from build123d import *

# Parameters (mm, degrees)
SKETCH_R        = 1.5
PAD_DEPTH       = 10
SKETCH001_R     = 4.5
POCKET_DEPTH    = 30.352032
SKETCH002_R     = 8.25
POCKET001_DEPTH = 25


with BuildPart() as part:
    # Sketch → Pad (new body)
    with BuildSketch(Plane.XY):
        with BuildLine():
            ThreePointArc((0, 70.5), (-15.559169, 68.761634), (-30.351032, 63.632263))
            Line((-30.351032, 63.632263), (-30.351032, 93.25))
            Line((-30.351032, 93.25), (0, 93.25))
            Line((0, 93.25), (0, 70.5))
        make_face()
        with Locations((-7.5, 90.25)):
            Circle(SKETCH_R, mode=Mode.SUBTRACT)
        with Locations((-22.5, 90.25)):
            Circle(SKETCH_R, mode=Mode.SUBTRACT)
    extrude(amount=PAD_DEPTH)

    # Sketch001 (on Face4 of Pad) → Pocket (cut, through all)
    with BuildSketch(Plane.YZ):
        with Locations((78.25, 0)):
            Circle(SKETCH001_R)
    extrude(amount=-POCKET_DEPTH, mode=Mode.SUBTRACT)

    # Sketch002 (on Face2 of Pocket) → Pocket001 (cut)
    with BuildSketch(Plane.YZ.offset(-2.5)):
        with Locations((78.25, 0)):
            Circle(SKETCH002_R)
    extrude(amount=-POCKET001_DEPTH, mode=Mode.SUBTRACT)


solid = part.part
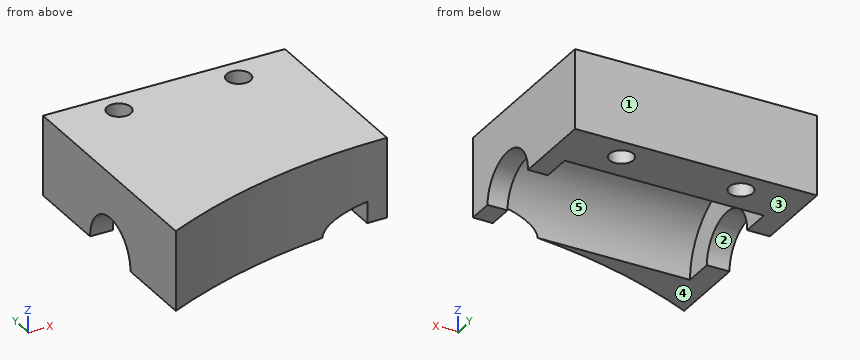
Can you work these out from the model? Positions are in its coordinate system, mm. Face numbers are marked on the shaded views. A direction names the side the tool comes from. Coordinates: 2 decimals unless noted, no trailing zeros. Write each loop counter-clockwise with the first axis right and the second up, starting at its lowest first coordinate (ties: lowest second). Pieces come first, ordered by that corner, then holes. Notation, with made-up numbers: (87.25, -20) -> (123.25, -20) arc R15 cw to (123.25, -1) -> close; hole circle Ø8 at (-17, 67). An arc over 180 degrees is marked (long way). Write each question's results on one line, items separated by ' | '. Start each with the question number.
Q1. We'd pull the mould along Y, two halves only. Please class the marked faces 1, 2 and 3: +Y half, -Y half, draft (parallel to the pull), parting line (faces both ways), or undercut.
Q2. Imagine slicing it at B-B (z = 2). Write out the boundary of the cut face in (x, y).
Q3. If I drill on probe 1 along X at (y, z) = (90.25, 4.5); probe 2 along Y at (x, z) = (-22.5, 4.25); probe 3 along Y at (x, z) = (-22.5, 5.25), over which ranges is the centre line in solid material (lowest first)?
Q4. Imagine slicing it at C-C (z = 9.25). Write out the boundary of the cut face in (x, y), then the cut area to 3 significant figures.
Q5. Imagine slicing it at A-A (x = -22.5). Write out the boundary of the cut face in (y, z), then the cut area to 3 significant figures.
Q6. On a 3-axis mill with a long thin cutter (end or side, diameter ignored), from which of +Z, -Z, +X, -X, +Y, -Y can I reach the whole of each face in a straight line? I mean the marked faces 4 and 5. Say none if no direction works.
Q7. Imagine slicing it at D-D (y = 72). Write out the boundary of the cut face in (x, z).
Q8. I'm going to push a flat-ended pin straight in: pin 1 (2 mm diameter, centred on x = -14, z = 2.5, fed in from -Y). Where does the tip first touch, or does it pass through?
Taken from the geometry:
1) face 1: +Y half | face 2: undercut | face 3: draft
2) outline: (-30.35, 63.63) arc R70.5 cw to (-5.98, 70.25) -> (-27.5, 70.25) -> (-27.5, 74.22) -> (-30.35, 74.22) -> close; (-30.35, 82.28) -> (-27.5, 82.28) -> (-27.5, 86.25) -> (-2.5, 86.25) -> (-2.5, 82.28) -> (0, 82.28) -> (0, 93.25) -> (-30.35, 93.25) -> close; (-2.5, 70.46) arc R70.5 cw to (0, 70.5) -> (0, 74.22) -> (-2.5, 74.22) -> close; hole circle Ø3 at (-22.5, 90.25); hole circle Ø3 at (-7.5, 90.25)
3) probe 1: x = -30.35 to -24, -21 to -9, -6 to 0 | probe 2: y = 66.81 to 71.18, 85.32 to 88.75, 91.75 to 93.25 | probe 3: y = 66.81 to 71.89, 84.61 to 88.75, 91.75 to 93.25
4) outline: (-30.35, 63.63) arc R70.5 cw to (0, 70.5) -> (0, 93.25) -> (-30.35, 93.25) -> close; hole circle Ø3 at (-22.5, 90.25); hole circle Ø3 at (-7.5, 90.25) | area: 744 mm^2
5) outline: (66.81, 0) -> (70, 0) arc R8.25 cw to (86.5, 0) -> (88.75, 0) -> (88.75, 10) -> (66.81, 10) -> close; (91.75, 0) -> (93.25, 0) -> (93.25, 10) -> (91.75, 10) -> close | area: 127 mm^2
6) face 4: -Z, +X, -X, +Y, -Y | face 5: -Z
7) outline: (-30.35, 0) -> (-27.5, 0) -> (-27.5, 5.39) -> (-2.5, 5.39) -> (-2.5, 0) -> (0, 0) -> (0, 10) -> (-30.35, 10) -> close
8) pin 1: stops at y = 68.89
